Geometry check sheet. Reference: drawing and pictorial views, mm from the part's lowest x, y, z. A direction names the side the tool comes from. Round coordinates to 2 decimals unless told otherwise and drop trailing zeros. Write each loop counter-clockwise with the first axis right and the second up, starting at its lowest first coordinate (ties: lowest second). Pieces come first, ordered by that corner, then holes. Notation, with made-up numbers: M 78,21 L 87,21 A21 ccw 87,49 Z; hole C -2,-27.5 d4. An arc over 180 degrees is marked long. Answer in a Markdown table with one row per item. Add a question column.
1. Go/stop test with flat-tipped pins: pin 1 Ø6 at (x, y) = (9.5, 9.5) entering from -Z; pin 2 Ø6 at (x, z) = (16.5, 8.5) entering from +Y; pin 3 Ø6 at (x, y) = (5.5, 15.5) entering from +Z (1 decimal). Record where each tip stops, or that it passes through.
2. Sectioned sample at D-D on z = 7.75. Record the cut outline in (x, y).
3. Set-up check for the marked faces 1, 2 and 3: record each of +Z, -Z, +X, -X, +Y, -Y from which the full face is reachable in a straight line by a thin tool's end or side.
4. Sectioned sample at B-B on x = 9.5. Record the cut outline in (y, z).
5. Sectioned sample at C-C on y = 1.5. Record the cut outline in (x, z).
6. Material ranges on probe 1 along Y at (x, z) = (9.5, 9.5) (1 decimal); probe 2 along Y at (x, z) = (8, 7.75) (1 decimal); probe 3 along X at (y, z) = (9.5, 9), recorded low to high.
7. Draft check along Y on the marked faces 4, 5 and 6. Enter one of: pulls with the +Y half, pulls with the -Y half, needs draft (parallel to the pull), parting line crosses it, or undercut.
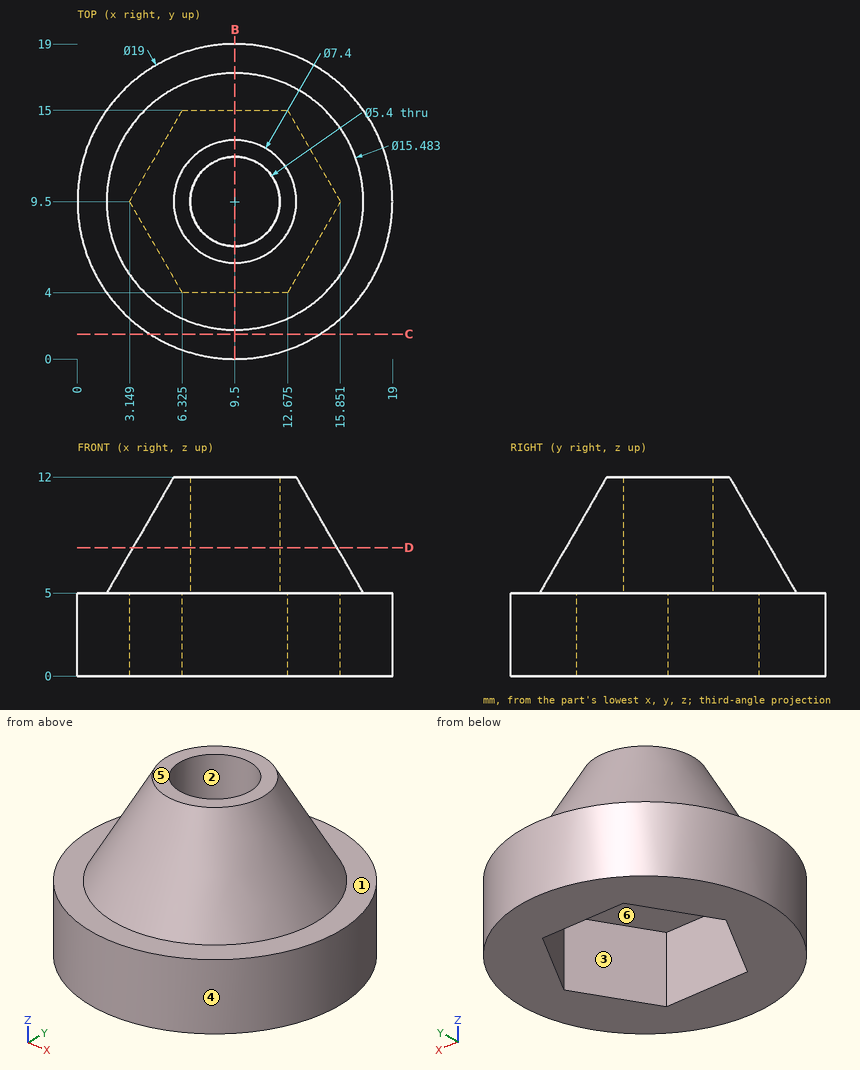
Geometry check:
| question | item | result |
|---|---|---|
| 1 | pin 1 | stops at z = 5 |
| 1 | pin 2 | stops at y = 14.46 |
| 1 | pin 3 | stops at z = 11.1 |
| 2 | outline | C 9.5,9.5 d12.31; hole C 9.5,9.5 d5.4 |
| 3 | face 1 | +Z |
| 3 | face 2 | +Z, -Z |
| 3 | face 3 | -Z |
| 4 | outline | M 0,0 L 4,0 L 4,5 L 6.8,5 L 6.8,12 L 5.8,12 L 1.76,5 L 0,5 Z; M 12.2,5 L 15,5 L 15,0 L 19,0 L 19,5 L 17.24,5 L 13.2,12 L 12.2,12 Z |
| 5 | outline | M 4.38,0 L 14.62,0 L 14.62,5 L 4.38,5 Z |
| 6 | probe 1 | y = 4.4 to 6.8, 12.2 to 14.6 |
| 6 | probe 2 | y = 3.5 to 7.3, 11.7 to 15.5 |
| 6 | probe 3 | x = 4.07 to 6.8, 12.2 to 14.93 |
| 7 | face 4 | parting line crosses it |
| 7 | face 5 | needs draft |
| 7 | face 6 | undercut |
